from build123d import *

# Parameters (mm, degrees)
ESQUISSE1_W                  = 20
ESQUISSE1_H                  = 192
BOSS_EXTRU_1_DEPTH           = 6
ENL_V_MAT_EXTRU_1_DEPTH      = 194.132079158
ENL_V_MAT_EXTRU_1_DEPTH_BACK = 194.132079158
ESQUISSE2_R                  = 4
CONG_1_R                     = 10
CONG_2_R                     = 5
ENL_V_MAT_EXTRU_2_DEPTH      = 194.132079158
ENL_V_MAT_EXTRU_2_DEPTH_BACK = 194.132079158
ESQUISSE3_R                  = 1.25


with BuildPart() as part:
    # Esquisse1 → Boss.-Extru.1 (new body)
    with BuildSketch(Plane.XY):
        with Locations((10, 96)):
            Rectangle(ESQUISSE1_W, ESQUISSE1_H)
    extrude(amount=BOSS_EXTRU_1_DEPTH)

    # Esquisse2 → Enlèv. mat.-Extru.1 (cut, two sides: drawn at the far end of the back side and taken through both)
    with BuildSketch(Plane.XY.offset(6).offset(-ENL_V_MAT_EXTRU_1_DEPTH_BACK)):
        with Locations((10, 10)):
            Circle(ESQUISSE2_R)
    extrude(amount=ENL_V_MAT_EXTRU_1_DEPTH + ENL_V_MAT_EXTRU_1_DEPTH_BACK, mode=Mode.SUBTRACT)

    # Congé1
    cong_1_edges = [part.edges().sort_by_distance(p)[0] for p in [
        (20, 0, 3),
        (0, 0, 3),
    ]]
    fillet(cong_1_edges, radius=CONG_1_R - 0.0001)  # a hair under: the kernel refuses the full size

    # Congé2
    cong_2_edges = [part.edges().sort_by_distance(p)[0] for p in [
        (0, 192, 3),
        (20, 192, 3),
    ]]
    fillet(cong_2_edges, radius=CONG_2_R)

    # Esquisse3 → Enlèv. mat.-Extru.2 (cut, two sides: drawn at the far end of the back side and taken through both)
    with BuildSketch(Plane.XY.offset(6).offset(-ENL_V_MAT_EXTRU_2_DEPTH_BACK)):
        with Locations((10, 17)):
            Circle(ESQUISSE3_R)
        with Locations((17, 10)):
            Circle(ESQUISSE3_R)
        with Locations((10, 3)):
            Circle(ESQUISSE3_R)
        with Locations((3, 10)):
            Circle(ESQUISSE3_R)
    extrude(amount=ENL_V_MAT_EXTRU_2_DEPTH + ENL_V_MAT_EXTRU_2_DEPTH_BACK, mode=Mode.SUBTRACT)


solid = part.part
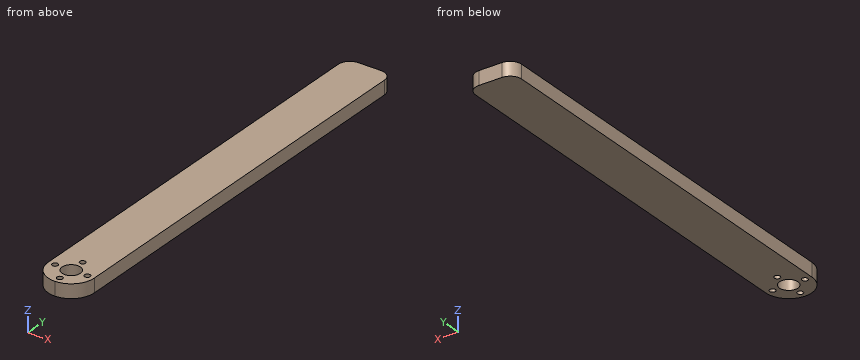
Verification items for the finished model (mm, model axes). Give positions to 0.01 mm unless a question says otherwise; leave off trailing zeros.
1) Depth check by flat-ended pin: pin 1 Ø2 at (x, z) = (14.5, 3) entering from -Y. Enter the tip coordinate at first touch or a pass-through.
2) Sectioned sample at A-A, the plane z = 3. Count the separate pieces of the cut face and the enclosed holes in it, then the cut area to 3 significant figures.
3) Thickness scan on line 1 along X through (y, z) = (10, 3.3); line 2 along Y through (x, z) = (10, 3.35); line 3 along X through (y, z) = (17, 3.5). Record the ranges inside material, lowest first.
Answers:
1. pin 1: stops at y = 0.63
2. separate pieces: 1
2. enclosed holes: 5
2. area: 3,720 mm2
3. line 1: x = 0 to 1.75, 4.25 to 6, 14 to 15.75, 18.25 to 20
3. line 2: y = 0 to 1.75, 4.25 to 6, 14 to 15.75, 18.25 to 192
3. line 3: x = 0 to 8.75, 11.25 to 20
